```python
from build123d import *

# Parameters (mm, degrees)
F0_W     = 78.2610476017
F0_H     = 61.8856586516
F1_DEPTH = 56.134
F4_R     = 7.271205843
F5_DEPTH = 56.642


# Not quite as in the source:
# - the program builds the solid bodies; features that only make, move or delete a surface that nothing else refers to are left out


with BuildPart() as f1:
    # F0 (on Right) → F1 (new body)
    with BuildSketch(Plane.YZ):
        with Locations((39.1305238008, -30.9428293258)):
            Rectangle(F0_W, F0_H)
    extrude(amount=F1_DEPTH)

    # F4 (on face) → F5 (join)
    with BuildSketch(Plane.XY):
        with Locations((27.1040890366, 40.5922196805)):
            Circle(F4_R)
        with BuildLine():
            ThreePointArc((24.2466891936, 14.9025116275), (26.8248957449, 14.6298549046), (28.1992270717, 16.8281961232))
            ThreePointArc((28.1992270717, 16.8281961232), (27.3655770879, 18.6672690129), (25.4330261647, 19.2524256742))
            ThreePointArc((25.4330261647, 19.2524256742), (24.2724174076, 17.232224668), (24.2466891936, 14.9025116275))
        make_face()
        with BuildLine():
            ThreePointArc((25.4330261647, 19.2524256742), (27.3655770879, 18.6672690129), (28.1992270717, 16.8281961232))
            ThreePointArc((28.1992270717, 16.8281961232), (26.8248957449, 14.6298549046), (24.2466891936, 14.9025116275))
            ThreePointArc((24.2466891936, 14.9025116275), (29.2863202966, 11.4378625234), (33.3389067896, 16.0180609673))
            ThreePointArc((33.3389067896, 16.0180609673), (30.4716460582, 20.2890111986), (25.4330261647, 19.2524256742))
        make_face()
        with BuildLine():
            ThreePointArc((24.2466891936, 14.9025116275), (24.2724174076, 17.232224668), (25.4330261647, 19.2524256742))
            ThreePointArc((25.4330261647, 19.2524256742), (23.394656757, 17.4716132859), (24.2466891936, 14.9025116275))
        make_face()
    extrude(amount=F5_DEPTH)


solid = f1.part
```
Model file for the job. Use its own axes, mm. A direction names the side the tool comes from. Coordinates: 2 decimals unless noted, no trailing zeros. Loops run counter-clockwise (first coordinate to the right, second up) from the corner with the lowest first, then second, coordinate; pieces in that order, holes last. Notation, with made-up numbers: (-22, -39.75) - (33, -39.75) arc R13 ccw to (33, -26.75) - close; hole circle Ø10 at (79.5, 58). An arc over 180 degrees is marked (long way). Answer as a JSON object with one key per item and string values. Group by question number.
(1) Two-plate mould, pull along Y, no slides. Class faces 1 (the face through (28, 0, -31)), 2 (the face through (0, 39, -31)), 3 (the face through (21.745, 45.506, 27.925)): released by +Y, released by -Y, zero draft, split by the parting line, or undercut.
(2) Flat gauge pin, fed straight in: pin 1 (5 mm diameter, centred on x = 9.5, y = 26, fed in from +Z). Where does the tip first touch, or does it go through?
(3) Cut at A-A (z = 17). Give the cut face in (x, y).
(4) Cut at D-D (y = 72.5). Give the cut face in (x, z), then the cut area to 3 significant figures.
(5) Cut at C-C (x = 31). Give the cut face in (y, z), then the cut area to 3 significant figures.
(6) Cut at B-B (y = 45). Give the cut face in (x, z), then the cut area to 3 significant figures.
(7) Probe line 1 along Z through (x, y) = (50.5, 56.5); line 2 along X through (y, z) = (14, 48); line 3 along X through (y, z) = (14.5, 50). List the from-to ranges inside material, lowest first.
(8) Tool access for faces 4 (the face through (27, 41, 56.642)), 5 (the face through (23.406, 17.51, 27.925)), 6 (the face through (28, 30, 0)): list every direction of +Z, -Z, +X, -X, +Y, -Y with a clear straight run to the whole face (end or side of a thin tool).
Geometry says:
{
 "1": {"face 1": "released by -Y", "face 2": "zero draft", "face 3": "undercut"},
 "2": {"pin 1": "stops at z = 0"},
 "3": {"outline": "circle Ø14.54 at (27.1, 40.59); (24.25, 14.9) arc R4.61 ccw (long way) to (25.43, 19.25) arc R2.45 ccw to start"},
 "4": {"outline": "(0, -61.89) - (56.13, -61.89) - (56.13, 0) - (0, 0) - close", "area": "3,470 mm^2"},
 "5": {"outline": "(0, -61.89) - (78.26, -61.89) - (78.26, 0) - (46.73, 0) - (46.73, 56.64) - (34.45, 56.64) - (34.45, 0) - (20.03, 0) - (20.03, 56.64) - (12, 56.64) - (12, 0) - (0, 0) - close", "area": "5,990 mm^2"},
 "6": {"outline": "(0, -61.89) - (56.13, -61.89) - (56.13, 0) - (32.89, 0) - (32.89, 56.64) - (21.32, 56.64) - (21.32, 0) - (0, 0) - close", "area": "4,130 mm^2"},
 "7": {"line 1": "z = -61.89 to 0", "line 2": "x = 24.57 to 32.87", "line 3": "x = 24.37 to 33.08"},
 "8": {"face 4": "+Z, +X, -X, +Y, -Y", "face 5": "+Z, -X", "face 6": "+Z"}
}
